Input: part model. Units: mm. Frame: model coordinates. Face numbers are marked on the shaded views. A direction names the side the tool comes from. Round coordinates to 2 decimals unless told otherwise and drop trailing zeros. Order: outer loops, then holes, each group sorted by start corner. A loop starts at its lowest first (then second) coordinate and runs counter-clockwise, first axis right, second up. Notation, with made-up numbers: (33, 18.25) -> (67, 18.25) arc R24 ccw to (67, 37.25) -> close; hole circle Ø2 at (38, -37.75). An arc over 180 degrees is marked (long way). Use a Markdown table: item, result.
from build123d import *

# Parameters (mm, degrees)
SKETCH_R           = 15
PAD_DEPTH          = 10
SKETCH001_R        = 11
POCKET_DEPTH       = 5
SKETCH002_R        = 7.5
PAD001_DEPTH       = 30
SKETCH003_R        = 1.25
POCKET001_DEPTH    = 3
POLARPATTERN_COUNT = 4
SKETCH004_R        = 4
POCKET002_DEPTH    = 10
POCKET003_DEPTH    = 2.5
FILLET_R           = 1
CHAMFER_ANGLE      = 45
CHAMFER_SIZE       = 1
CHAMFER001_ANGLE   = 45
CHAMFER001_SIZE    = 1


with BuildPart() as part:
    # Sketch → Pad (new body)
    with BuildSketch(Plane.YZ):
        Circle(SKETCH_R)
    extrude(amount=PAD_DEPTH)

    # Sketch001 (on Face3 of Pad) → Pocket (cut)
    with BuildSketch(Plane.YZ.offset(10)):
        Circle(SKETCH001_R)
    extrude(amount=-POCKET_DEPTH, mode=Mode.SUBTRACT)

    # Sketch002 (on Face2 of Pocket) → Pad001 (join)
    with BuildSketch(Plane(origin=(0, 0, 0), x_dir=(0, 1, 0), z_dir=(-1, 0, 0))):
        Circle(SKETCH002_R)
    extrude(amount=PAD001_DEPTH)

    # Sketch003 (on Face3 of Pad001) → Pocket001 (cut)
    with BuildSketch(Plane.YZ.offset(10)):
        with Locations((0, 13)):
            Circle(SKETCH003_R)
    pocket001 = extrude(amount=-POCKET001_DEPTH, mode=Mode.SUBTRACT)

    # PolarPattern: Pocket001 ×4 about axis
    polarpattern_axis = Axis((10, 0, 0), (1, 0, 0))
    for i in range(1, POLARPATTERN_COUNT):
        add(pocket001.rotate(polarpattern_axis, i * 360 / POLARPATTERN_COUNT), mode=Mode.SUBTRACT)

    # Sketch004 (on Face10 of PolarPattern) → Pocket002 (cut)
    with BuildSketch(Plane(origin=(-30, 0, 0), x_dir=(0, 1, 0), z_dir=(-1, 0, 0))):
        Circle(SKETCH004_R)
    extrude(amount=-POCKET002_DEPTH, mode=Mode.SUBTRACT)

    # Sketch005 (on DatumPlane) → Pocket003 (cut, symmetric)
    with BuildSketch(Plane(origin=(-15, 7.5, 0), x_dir=(0, 0, -1), z_dir=(-0.087156, 0.996195, 0))):
        with BuildLine():
            ThreePointArc((3, 6.025), (0, 9.025), (-3, 6.025))
            Line((-3, 6.025), (-3, -6.025))
            ThreePointArc((-3, -6.025), (0, -9.025), (3, -6.025))
            Line((3, -6.025), (3, 6.025))
        make_face()
    extrude(amount=POCKET003_DEPTH, both=True, mode=Mode.SUBTRACT)

    # Fillet
    fillet_edges = [part.edges().sort_by_distance(p)[0] for p in [
        (10, -15, 0),
    ]]
    fillet(fillet_edges, radius=FILLET_R)

    # Chamfer
    chamfer_edges = [part.edges().sort_by_distance(p)[0] for p in [
        (0, -15, 0),
    ]]
    chamfer_side = part.faces().sort_by_distance((4.520615, -15, 0))[0]
    chamfer(chamfer_edges, length=CHAMFER_SIZE, angle=CHAMFER_ANGLE, reference=chamfer_side)

    # Chamfer001
    chamfer001_edges = [part.edges().sort_by_distance(p)[0] for p in [
        (-30, -7.5, 0),
    ]]
    chamfer001_side = part.faces().sort_by_distance((-15, -7.5, 0))[0]
    chamfer(chamfer001_edges, length=CHAMFER001_SIZE, angle=CHAMFER001_ANGLE, reference=chamfer001_side)


solid = part.part
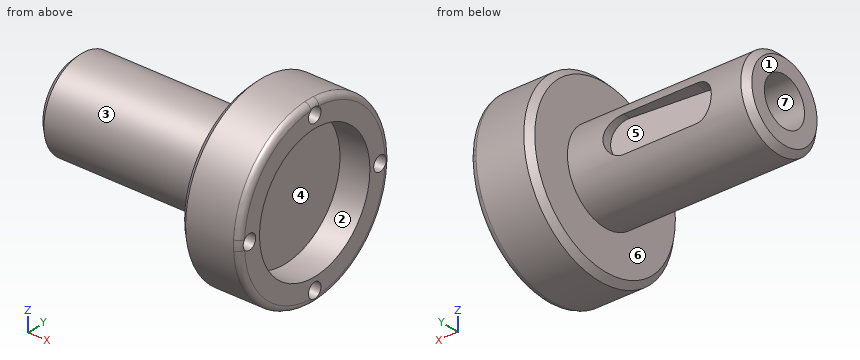
1) Draft query along X for the marked faces 4, 5, 6 and 7. Return one class per face: released by +X, released by -X, zero draft, split by the parting line, or undercut.
Answer key:
| item | result |
|---|---|
| face 4 | released by +X |
| face 5 | undercut |
| face 6 | released by -X |
| face 7 | zero draft |
2) Contact query for flat-ended pins moving along their axis: P1, Ø2, axis at y = 0, z = 13, coming from the +X side; P2, Ø6.5, axis at y = -4, z = -1.5, coming from the +X side; P3, Ø3, axis at x = 0.5, z = 4, coming from the -Y side. Output: stop coordinate, or through.
Answer key:
| item | result |
|---|---|
| P1 | stops at x = 7 |
| P2 | stops at x = 5 |
| P3 | stops at y = -14.78 |
3) Ray query, probe 1 along Z at (x, y) = (8, 0); probe 2 along Z at (x, y) = (-23, 0). Return the intervals inside material, ascending.
Answer key:
| item | result |
|---|---|
| probe 1 | z = -15 to -14.25, -11.75 to -11, 11 to 11.75, 14.25 to 15 |
| probe 2 | z = -7.5 to -4, 4 to 7.5 |
4) Cut plane A-A on x = 5.5. Return loops of the section in (y, z), and give its area (3 significant figures).
Answer key:
| item | result |
|---|---|
| outline | circle Ø30 at (0, 0); hole circle Ø22 at (0, 0) |
| area | 327 mm^2 |
5) Cut plane B-B on x = -15.5. Return loops of the section in (y, z).
Answer key:
| item | result |
|---|---|
| outline | (4.95, -3) -> (4.95, 3) -> (6.87, 3) arc R7.5 ccw (long way) to (6.87, -3) -> close |
6) Set-up query: the marked faces 1, 2 and 3. Return all of +Z, -Z, +X, -X, +Y, -Y with unobstructed straight access to the full face (end or side cutting, diameter ignored); none if empty.
Answer key:
| item | result |
|---|---|
| face 1 | +Z, -Z, -X, +Y, -Y |
| face 2 | +X |
| face 3 | -X |
